Input: part model. Units: mm. Frame: model coordinates. A direction names the side the tool comes from. Coordinates: 2 decimals unless noted, no trailing zeros. Order: outer loops, then holes, each group sorted by start corner. A loop starts at its lowest first (then second) coordinate and runs counter-clockwise, first axis right, second up.
from build123d import *

# Parameters (mm, degrees)
ESQUISSE1_W             = 50
ESQUISSE1_H             = 50
BOSS_EXTRU_1_DEPTH      = 7
CHANFREIN1_SIZE         = 10
BOSS_EXTRU_2_DEPTH      = 40
BOSS_EXTRU_3_DEPTH      = 6
ESQUISSE5_R             = 11.25
ENL_V_MAT_EXTRU_1_DEPTH = 7
ESQUISSE6_R             = 2.5
ESQUISSE6_R_2           = 2.745007664
ENL_V_MAT_EXTRU_2_DEPTH = 6
ESQUISSE7_R             = 2
ENL_V_MAT_EXTRU_3_DEPTH = 7


with BuildPart() as part:
    # Esquisse1 → Boss.-Extru.1 (new body)
    with BuildSketch(Plane.XY):
        with Locations((-1.883571087, -2.012711864)):
            Rectangle(ESQUISSE1_W, ESQUISSE1_H)
    extrude(amount=BOSS_EXTRU_1_DEPTH)

    # Chanfrein1
    chanfrein1_edges = [part.edges().sort_by_distance(p)[0] for p in [
        (-26.883571087, 22.987288136, 3.5),
        (23.116428913, 22.987288136, 3.5),
        (23.116428913, -27.012711864, 3.5),
        (-26.883571087, -27.012711864, 3.5),
    ]]
    chamfer(chanfrein1_edges, length=CHANFREIN1_SIZE)

    # Esquisse2 → Boss.-Extru.2 (add)
    with BuildSketch(Plane.XY.offset(7)):
        Polygon((-23.348037181, 9.45175423), (-26.883571087, 12.987288136), (-16.883571087, 22.987288136), (-13.348037181, 19.45175423), align=None)
        Polygon((19.580895007, -13.477177958), (9.580895007, -23.477177958), (13.116428913, -27.012711864), (23.116428913, -17.012711864), align=None)
        Polygon((-13.348037181, -23.477177958), (-23.348037181, -13.477177958), (-26.883571087, -17.012711864), (-16.883571087, -27.012711864), align=None)
    extrude(amount=BOSS_EXTRU_2_DEPTH)

    # Esquisse4 → Boss.-Extru.3 (add)
    with BuildSketch(Plane.XY.offset(47)):
        Polygon((-18.348037181, 14.45175423), (-13.348037181, 19.45175423), (-16.883571087, 22.987288136), (-26.883571087, 12.987288136), (-26.883571087, -17.012711864), (-16.883571087, -27.012711864), (13.116428913, -27.012711864), (23.116428913, -17.012711864), (19.580895007, -13.477177958), (14.580895007, -18.477177958), (-18.348037181, -18.477177958), align=None)
    extrude(amount=BOSS_EXTRU_3_DEPTH)

    # Esquisse5 → Enlèv. mat.-Extru.1 (cut)
    with BuildSketch(Plane(origin=(0, 0, 0), x_dir=(-1, 0, 0), z_dir=(0, 0, -1))):
        with Locations((1.883571087, -2.012711864)):
            Circle(ESQUISSE5_R)
    extrude(amount=-ENL_V_MAT_EXTRU_1_DEPTH, mode=Mode.SUBTRACT)

    # Esquisse6 → Enlèv. mat.-Extru.2 (cut)
    with BuildSketch(Plane.XY.offset(53)):
        with Locations((-22.648037181, -2.012711864)):
            Circle(ESQUISSE6_R)
        with Locations((-1.883571087, -22.777177958)):
            Circle(ESQUISSE6_R_2)
    extrude(amount=-ENL_V_MAT_EXTRU_2_DEPTH, mode=Mode.SUBTRACT)

    # Esquisse7 → Enlèv. mat.-Extru.3 (cut)
    with BuildSketch(Plane(origin=(0, 0, 0), x_dir=(-1, 0, 0), z_dir=(0, 0, -1))):
        with Locations((1.883571087, 12.987288136)):
            Circle(ESQUISSE7_R)
        with Locations((-13.116428913, -2.012711864)):
            Circle(ESQUISSE7_R)
    extrude(amount=-ENL_V_MAT_EXTRU_3_DEPTH, mode=Mode.SUBTRACT)


solid = part.part
Item 1: Draft query along Y for faces 5 (the face through (-15.091, 21.195, 29.678)), 6 (the face through (-25.091, 11.195, 26.72)), 7 (the face through (-26.884, -2, 50)). Return one class per face: pulls with the +Y half, pulls with the -Y half, needs draft (parallel to the pull), parting line crosses it, or undercut.
Response values:
face 5: pulls with the +Y half
face 6: undercut
face 7: needs draft
Item 2: Ray query, probe 1 along Z at (x, y) = (3.5, 19); probe 2 along Z at (x, y) = (-24.5, -10); probe 3 along Y at (x, z) = (-18, 29). Return the intervals inside material, ascending.
Response values:
probe 1: z = 0 to 7
probe 2: z = 0 to 7, 47 to 53
probe 3: y = -25.9 to -18.83, 14.8 to 21.87
Item 3: Pin query (flat end, axial travel): pin 1 Ø10 at (x, z) = (9, 14.5) entering from +Y; pin 2 Ø4 at (x, z) = (14.5, 12) entering from +Y; pin 3 Ø1 at (y, z) = (-20.5, 29) entering from -X. Return the tip coordinate at first contact, or that it passes through.
Response values:
pin 1: stops at y = -19.06
pin 2: stops at y = -16.56
pin 3: stops at x = -23.9
Item 4: Cut plane D-D on x = -21.5. Return loops of the section in (y, z).
Response values:
outline: (-22.4, 0) - (18.37, 0) - (18.37, 53) - (0.21, 53) - (0.21, 47) - (11.3, 47) - (11.3, 7) - (-15.33, 7) - (-15.33, 47) - (-4.23, 47) - (-4.23, 53) - (-22.4, 53) - close
Item 5: Cut plane A-A on z = 34.5. Return loops of the section in (x, y), then the cut area to 3 significant figures.
Response values:
outline: (-26.88, -17.01) - (-16.88, -27.01) - (-13.35, -23.48) - (-23.35, -13.48) - close; (-26.88, 12.99) - (-23.35, 9.45) - (-13.35, 19.45) - (-16.88, 22.99) - close; (9.58, -23.48) - (13.12, -27.01) - (23.12, -17.01) - (19.58, -13.48) - close
area: 212 mm2
Item 6: Access query for faces 1 (the face through (-2.2, 9.4, 7)), 2 (the face through (11.324, -25.22, 26.72)), 3 (the face through (14.65, -18.41, 29.68)), 4 (the face through (-25.09, -15.22, 26.72)). Directions: +Z, -Z, +X, -X, +Y, -Y. A direction counts if a zero-diameter tool reaches every point of the face in a straight line with its end or side. Return the directions, or none.
Response values:
face 1: none
face 2: -Y
face 3: +Y
face 4: -X
Item 7: Cut plane C-C on z = 50.5. Return loops of the section in (x, y) (3 decimals), then the cut area to 3 significant figures.
Response values:
outline: (-26.884, -17.013) - (-16.884, -27.013) - (13.116, -27.013) - (23.116, -17.013) - (19.581, -13.477) - (14.581, -18.477) - (-18.348, -18.477) - (-18.348, 14.452) - (-13.348, 19.452) - (-16.884, 22.987) - (-26.884, 12.987) - close; hole circle Ø5 at (-22.648, -2.013); hole circle Ø5.49 at (-1.884, -22.777)
area: 635 mm2
Item 8: Cut plane B-B on y = 1.5. Return loops of the section in (x, z).
Response values:
outline: (-26.88, 0) - (-12.57, 0) - (-12.57, 7) - (-26.88, 7) - close; (-26.88, 47) - (-18.35, 47) - (-18.35, 53) - (-26.88, 53) - close; (8.8, 0) - (23.12, 0) - (23.12, 7) - (8.8, 7) - close
